from build123d import *

# Parameters (mm, degrees)
EXTRUDE001_DEPTH = 1
EXTRUDE_DEPTH    = 2
BOX_W            = 190
BOX_H            = 2
BOX_DEPTH        = 1


with BuildPart() as extrude001:
    # Sketch001 → Extrude001 (new body)
    with BuildSketch(Plane.XY):
        Polygon((-95, 0), (95, 0), (85, 61), (-85, 61), align=None)
    extrude(amount=EXTRUDE001_DEPTH)


with BuildPart() as extrude001_1:
    # Extrude001 placement: moved
    add(extrude001.part.moved(Location((0, 0, 2))))


with BuildPart() as extrude_body:
    # Sketch → Extrude (new body)
    with BuildSketch(Plane.XY):
        Polygon((-95, 0), (95, 0), (85, 61), (-85, 61), align=None)
    extrude(amount=EXTRUDE_DEPTH)


with BuildPart() as fusion:
    # Box → Box (new body)
    with BuildSketch(Plane(origin=(-95, -2, 2), x_dir=(1, 0, 0), z_dir=(0, 0, 1))):
        with Locations((95, 1)):
            Rectangle(BOX_W, BOX_H)
    extrude(amount=BOX_DEPTH)

    # Fusion: union Extrude001, Extrude body
    add(extrude001_1.part)
    add(extrude_body.part)


solid = fusion.part
The model under review builds one solid part; all positions refer to its coordinate system, in mm. Give positions to 0.01 mm unless a question says otherwise; leave off trailing zeros. Order: outer loops, then holes, each group sorted by start corner. A loop starts at its lowest first (then second) coordinate and runs counter-clockwise, first axis right, second up. Notation, with made-up numbers: M 38,32 L 67,32 A34 ccw 67,63 Z; hole C 84,31 d5. An arc over 180 degrees is marked long. Answer in a Markdown table with one row per item. Add a question column.
1. Add section A-A on x = -40.5. State the section outline as (y, z) points.
2. Add section C-C on y = 16. State the section outline as (x, z) points.
3. To check wall thickness, follow line 1 along Y through (x, z) = (79, 1.15); line 2 along X through (y, z) = (43.5, 0.4); line 3 along X through (y, z) = (27, 0.85). State the ranges of each line that lie inside material, in increasing order.
4. Add section B-B on z = 1.1. State the section outline as (x, y) points, plus the area to 3 significant figures.
5. For pin 1 Ø0.6 at (x, y) = (42, -1.5) entering from -Z; pin 2 Ø1 at (y, z) = (26, 0.5) entering from -X, all flat-tipped, find the tip position at first contact; note any pin that passes through.
The answers:
| question | item | result |
|---|---|---|
| 1 | outline | M -2,2 L 0,2 L 0,0 L 61,0 L 61,3 L -2,3 Z |
| 2 | outline | M -92.38,0 L 92.38,0 L 92.38,3 L -92.38,3 Z |
| 3 | line 1 | 0 to 61 |
| 3 | line 2 | -87.87 to 87.87 |
| 3 | line 3 | -90.57 to 90.57 |
| 4 | outline | M -95,0 L 95,0 L 85,61 L -85,61 Z |
| 4 | area | 11,000 mm2 |
| 5 | pin 1 | z = 2 |
| 5 | pin 2 | x = -90.82 |
